Model file for the job. Use its own axes, mm. A direction names the side the tool comes from. Give positions to 0.01 mm unless a question says otherwise; leave off trailing zeros. Loops run counter-clockwise (first coordinate to the right, second up) from the corner with the lowest first, then second, coordinate; pieces in that order, holes last. Notation, with made-up numbers: M 75.5,-30.75 L 123.5,-30.75 A15 cw 123.5,-22.75 Z; hole C 7,87 d10. An arc over 180 degrees is marked long. Use CSV: the item, a comma, the result in double quotes. Start each with the question number.
(1) Flat gauge pins, fed straight in: P1, Ø1, axis at x = -279.5, y = -2.5, coming from the +Z side; P2, Ø6, axis at x = -65.5, y = -6, coming from the -Z side; P3, Ø8, axis at x = -48.5, z = 85, coming from the -Y side; P4, Ø1, axis at x = -114, y = -6.5, coming from the -Z side. Where does each tip first touch, or does it go through?
(2) Slice it at B-B on z = 72.5. List the corners of the cut face in (x, y), and give its area (3 significant figures).
(3) Slice it at D-D on z = 50. List the corners of the cut face in (x, y).
(4) Two-plate mould, pull along Z, no slides. Class faces 1 (the face through (-258.12, -4.93, 163.91)), 2 (the face through (-295.23, -4.93, 51.5)), 3 (the face through (-151, -5, 125.234)): pulls with the +Z half, pulls with the -Z half, needs draft (parallel to the pull), parting line crosses it, or undercut.
(5) Slice it at C-C on y = -1.5. State how many separate pieces and enclosed holes the cut face has, and give its area (3 significant figures).
(6) Wall check: line 1 along X through (y, z) = (-8, 54.5); line 2 along X through (y, z) = (-3.5, 48.5); line 3 along X through (y, z) = (-8.5, 44). Give the ranges that are in metal, low to high. Write a range as from..to.
(7) Tool access for faces 4 (the face through (-151.084, -4.93, 145.353)), 5 (the face through (-67.705, -4.93, 121.597)): list every direction of +Z, -Z, +X, -X, +Y, -Y with a clear straight run to the whole face (end or side of a thin tool).
(8) Slice it at A-A on x = -150. List the corners of the cut face in (y, z).
```python
from build123d import *

# Parameters (mm, degrees)
F0_R     = 5
F1_DEPTH = 10


with BuildPart() as f1:
    # F0 (on Front) → F1 (new body)
    with BuildSketch(Plane.XZ):
        with BuildLine():
            ThreePointArc((-219.160475, 174.812716), (-258.617076, 163.603922), (-286.288055, 133.32559))
            Line((-286.288055, 133.32559), (-322.419221, 61.063257))
            ThreePointArc((-322.419221, 61.063257), (-311.180493, 27.639014), (-277.697862, 38.702578))
            Line((-277.697862, 38.702578), (-277.580779, 38.936743))
            Line((-277.580779, 38.936743), (-242.002863, 111.033879))
            ThreePointArc((-242.002863, 111.033879), (-232.608699, 121.394639), (-219.160475, 125.234029))
            Line((-219.160475, 125.234029), (-80.808, 125.234029))
            ThreePointArc((-80.808, 125.234029), (-67.537861, 121.495487), (-58.170905, 111.37949))
            ThreePointArc((-58.170905, 111.37949), (-58.070965, 111.181769), (-57.972752, 110.983184))
            Line((-57.972752, 110.983184), (-21.891489, 38.820657))
            ThreePointArc((-21.891489, 38.820657), (11.086202, 28.061196), (21.985722, 60.992861))
            Line((21.985722, 60.992861), (-13.81966, 133.54102))
            ThreePointArc((-13.81966, 133.54102), (-41.346483, 163.59247), (-80.52456, 174.812716))
            Line((-80.52456, 174.812716), (-219.160475, 174.812716))
        make_face()
        with Locations((-300, 50)):
            Circle(F0_R, mode=Mode.SUBTRACT)
        with Locations((0, 50)):
            Circle(F0_R, mode=Mode.SUBTRACT)
        with Locations((-150, 150.234029)):
            Circle(F0_R, mode=Mode.SUBTRACT)
    extrude(amount=F1_DEPTH)


solid = f1.part
```
Reply:
1,P1,"stops at z = 145.06"
1,P2,"stops at z = 117.45"
1,P3,"stops at y = -10"
1,P4,"stops at z = 125.23"
2,outline,"M -316.7,-10 L -261.02,-10 L -261.02,0 L -316.7,0 Z; M -38.73,-10 L 16.31,-10 L 16.31,0 L -38.73,0 Z"
2,area,"1,110 mm^2"
3,outline,"M -325,-10 L -305,-10 L -305,0 L -325,0 Z; M -295,-10 L -272.12,-10 L -272.12,0 L -295,0 Z; M -27.48,-10 L -5,-10 L -5,0 L -27.48,0 Z; M 5,-10 L 24.58,-10 L 24.58,0 L 5,0 Z"
4,face 1,"pulls with the +Z half"
4,face 2,"undercut"
4,face 3,"pulls with the -Z half"
5,separate pieces,"1"
5,enclosed holes,"3"
5,area,"22,100 mm^2"
6,line 1,"x = -324.59..-302.18, -297.82..-269.9, -29.73..-2.18, 2.18..24.17"
6,line 2,"x = -324.96..-304.77, -295.23..-272.86, -26.73..-4.77, 4.77..24.53"
6,line 3,"x = -324.27..-275.08, -24.48..23.84"
7,face 4,"+Y, -Y"
7,face 5,"-Z, +Y, -Y"
8,outline,"M -10,125.23 L 0,125.23 L 0,145.23 L -10,145.23 Z; M -10,155.23 L 0,155.23 L 0,174.81 L -10,174.81 Z"
